Here's how the part is built. I have some questions about the finished solid (model axes, mm). A direction names the side the tool comes from. Coordinates: 2 decimals unless noted, no trailing zeros. Write each loop counter-clockwise with the first axis right and the second up, starting at its lowest first coordinate (ties: lowest second). Pieces come first, ordered by that corner, then holes. Notation, with made-up numbers: M 13,6.5 L 37,6.5 A17 cw 37,31.5 Z; hole C -3,8.25 d4. An arc over 180 degrees is marked long. Use one line per item in the form item = value. Start each with the question number.
1. I want a section at C-C, the plane y = 12.5. List the corners of the cut face in (x, z) for me.
2. Thinking about a two-plate mould opening in X: for faces 3 (the face through (15.1, 13.48, 2.35)), 4 (the face through (-10.82, -48.724, 2.348)), 5 (the face through (-15.18, 13.97, 2.35)), 6 (the face through (-1, 12, 4.762)), which applies, released by +X, released by -X, zero draft, split by the parting line, or undercut?
3. I want a section at D-D, the plane z = 1.2. List the corners of the cut face in (x, y) for me, plus the area to 3 significant figures.
4. On a 3-axis mill with a long thin cutter (end or side, diameter ignored), from which of +Z, -Z, +X, -X, +Y, -Y can I reach the whole of each face in a straight line? I mean faces 1 (the face through (0.12, 6.35, 2.35)), 2 (the face through (-1, 12, 0)). Say none if no direction works.
5. I want a section at A-A, the plane x = 0. List the corners of the cut face in (y, z) for me.
6. I want a section at B-B, the plane y = -29. List the corners of the cut face in (x, z) for me.
7. Please list where these lines run through material, in increasing order: line 1 along Y through (x, z) = (0, 2.15); line 2 along X through (y, z) = (12, 2.85); line 3 along X through (y, z) = (8.5, 1.45). Write a range as [from, to].
8. I'm going to push flat-ended pins straight in: pin 1 Ø2 at (x, z) = (-15, 2.5) entering from -Y; pin 2 Ø2 at (y, z) = (29, 3) entering from -X; pin 3 Ø8 at (x, y) = (-15.5, -34.5) entering from -Z; pin 4 Ø2 at (y, z) = (-14, 1.5) entering from -X. Where does each tip first touch, or does it pass through?
from build123d import *

# Parameters (mm, degrees)
F0_R     = 49.911
F0_R_2   = 6.35
F1_DEPTH = 4.7625
F3_DEPTH = 9.144


with BuildPart() as f1:
    # F0 (on Top) → F1 (new body)
    with BuildSketch(Plane.XY):
        Circle(F0_R)
        Circle(F0_R_2, mode=Mode.SUBTRACT)
    extrude(amount=F1_DEPTH)

    # F2 (on face) → F3 (cut)
    with BuildSketch(Plane(origin=(0, 0, 0), x_dir=(1, 0, 0), z_dir=(0, 0, -1))):
        with BuildLine():
            ThreePointArc((25.7526882864, -22.9879649836), (32.253966126, -12.3015916531), (34.5202475087, 0))
            ThreePointArc((34.5202475087, 0), (-12.546596424, 32.1594528286), (-25.3999721233, -23.3771021343))
            Line((-25.3999721233, -23.3771021343), (-4.6723252185, -4.3002182564))
            ThreePointArc((-4.6723252185, -4.3002182564), (-2.3079465833, 5.9157317864), (6.35, 0))
            ThreePointArc((6.35, 0), (5.9331175088, -2.2628779524), (4.7372073615, -4.2286364722))
            Line((4.7372073615, -4.2286364722), (25.7526882864, -22.9879649836))
        make_face()
    extrude(amount=-F3_DEPTH, mode=Mode.SUBTRACT)


solid = f1.part
Answer list:
q1.outline = M -48.32,0 L -32.18,0 L -32.18,4.76 L -48.32,4.76 Z; M -13.58,0 L 14,0 L 14,4.76 L -13.58,4.76 Z; M 32.18,0 L 48.32,0 L 48.32,4.76 L 32.18,4.76 Z
q2.face_3 = undercut
q2.face_4 = split by the parting line
q2.face_5 = undercut
q2.face_6 = zero draft
q3.outline = C 0,0 d99.82; hole M -25.4,23.38 A34.52 ccw long 25.75,22.99 L 4.74,4.23 A6.35 ccw -4.67,4.3 Z
q3.area = 5,040 mm²
q4.face_1 = +Z, -Z
q4.face_2 = -Z, +X, -X, +Y, -Y
q5.outline = M -49.91,0 L -34.52,0 L -34.52,4.76 L -49.91,4.76 Z; M 6.35,0 L 49.91,0 L 49.91,4.76 L 6.35,4.76 Z
q6.outline = M -40.62,0 L -18.73,0 L -18.73,4.76 L -40.62,4.76 Z; M 18.73,0 L 40.62,0 L 40.62,4.76 L 18.73,4.76 Z
q7.line_1 = [-49.91, -34.52], [6.35, 49.91]
q7.line_2 = [-48.45, -32.37], [-13.04, 13.44], [32.37, 48.45]
q7.line_3 = [-49.18, -33.46], [-9.24, 9.52], [33.46, 49.18]
q8.pin_1 = -47.91
q8.pin_2 = -41.32
q8.pin_3 = 0
q8.pin_4 = -48.19
